The model under review builds one solid part; all positions refer to its coordinate system, in mm. A direction names the side the tool comes from. Coordinates: 2 decimals unless noted, no trailing zeros. Loops run counter-clockwise (first coordinate to the right, second up) from the corner with the lowest first, then second, coordinate; pieces in that order, holes last. Notation, with made-up numbers: (84.25, 60) -> (103.25, 60) arc R5 ccw to (103.25, 66) -> close; hole circle Ø6 at (9, -7.5). An arc over 180 degrees is marked (long way). One line per question, with ' | ' between items. Start each with the question number.
from build123d import *

# Parameters (mm, degrees)
F0_W        = 110
F0_H        = 110
F0_R        = 7
F0_R_2      = 6.6
F0_R_3      = 4.5
F0_R_4      = 5.5
F1_DEPTH    = 20
F2_DEPTH    = 20.001
F3_DEPTH    = 8
F4_DEPTH    = 9.4
F5_SIZE     = 1
F6_T1_DEPTH = 133.7168298797
F6_T3_DEPTH = 133.7168298797
F7_SIZE     = 0.5


# Not quite as in the source:
# - a fillet or chamfer that OpenCascade refuses, or shapes differently, is made with other operations: its cross-section is extruded or revolved along the edge and cut away or added


with BuildPart() as f1:
    # F0 (on Right) → F1 (new body)
    with BuildSketch(Plane.YZ):
        Rectangle(F0_W, F0_H)
        with Locations((-42.4264068712, -42.4264068712)):
            Circle(F0_R, mode=Mode.SUBTRACT)
        with Locations((42.4264068712, -42.4264068712)):
            Circle(F0_R, mode=Mode.SUBTRACT)
        with Locations((-42.4264068712, 42.4264068712)):
            Circle(F0_R, mode=Mode.SUBTRACT)
        Circle(F0_R_2, mode=Mode.SUBTRACT)
        with Locations((42.4264068712, 42.4264068712)):
            Circle(F0_R, mode=Mode.SUBTRACT)
        with Locations((-42.4264068712, 42.4264068712)):
            Circle(F0_R)
        with Locations((-42.4264068712, 42.4264068712)):
            Circle(F0_R_3, mode=Mode.SUBTRACT)
        with Locations((-42.4264068712, -42.4264068712)):
            Circle(F0_R)
        with Locations((-42.4264068712, -42.4264068712)):
            Circle(F0_R_3, mode=Mode.SUBTRACT)
        with Locations((42.4264068712, -42.4264068712)):
            Circle(F0_R)
        with Locations((42.4264068712, -42.4264068712)):
            Circle(F0_R_3, mode=Mode.SUBTRACT)
        with Locations((42.4264068712, 42.4264068712)):
            Circle(F0_R)
        with Locations((42.4264068712, 42.4264068712)):
            Circle(F0_R_3, mode=Mode.SUBTRACT)
        Circle(F0_R_2)
        Circle(F0_R_4, mode=Mode.SUBTRACT)
        Circle(F0_R_4)
        with Locations((-42.4264068712, 42.4264068712)):
            Circle(F0_R_3)
        with Locations((-42.4264068712, -42.4264068712)):
            Circle(F0_R_3)
        with Locations((42.4264068712, -42.4264068712)):
            Circle(F0_R_3)
        with Locations((42.4264068712, 42.4264068712)):
            Circle(F0_R_3)
    extrude(amount=-F1_DEPTH)

    # F0 (on Right) → F2 (cut, through all)
    with BuildSketch(Plane.YZ):
        with Locations((-42.4264068712, 42.4264068712)):
            Circle(F0_R_3)
        with Locations((42.4264068712, -42.4264068712)):
            Circle(F0_R_3)
        with Locations((-42.4264068712, -42.4264068712)):
            Circle(F0_R_3)
        Circle(F0_R_4)
        with Locations((42.4264068712, 42.4264068712)):
            Circle(F0_R_3)
    extrude(amount=-F2_DEPTH, mode=Mode.SUBTRACT)

    # F0 (on Right) → F3 (cut)
    with BuildSketch(Plane.YZ):
        with Locations((-42.4264068712, 42.4264068712)):
            Circle(F0_R)
        with Locations((-42.4264068712, 42.4264068712)):
            Circle(F0_R_3, mode=Mode.SUBTRACT)
        with Locations((42.4264068712, 42.4264068712)):
            Circle(F0_R)
        with Locations((42.4264068712, 42.4264068712)):
            Circle(F0_R_3, mode=Mode.SUBTRACT)
        with Locations((-42.4264068712, -42.4264068712)):
            Circle(F0_R)
        with Locations((-42.4264068712, -42.4264068712)):
            Circle(F0_R_3, mode=Mode.SUBTRACT)
        with Locations((42.4264068712, -42.4264068712)):
            Circle(F0_R)
        with Locations((42.4264068712, -42.4264068712)):
            Circle(F0_R_3, mode=Mode.SUBTRACT)
    extrude(amount=-F3_DEPTH, mode=Mode.SUBTRACT)

    # F0 (on Right) → F4 (cut)
    with BuildSketch(Plane.YZ):
        Circle(F0_R_2)
        Circle(F0_R_4, mode=Mode.SUBTRACT)
    extrude(amount=-F4_DEPTH, mode=Mode.SUBTRACT)

    # F5
    f5_edges = [f1.edges().sort_by_distance(p)[0] for p in [
        (0, -49.426407, 42.426407),
        (0, 35.426407, 42.426407),
        (0, -49.426407, -42.426407),
        (0, 35.426407, -42.426407),
        (-10, 55, -55),
        (-10, 55, 55),
        (-10, -55, 55),
        (-10, -55, -55),
    ]]
    chamfer(f5_edges, length=F5_SIZE)

    # F6: chamfer of 5 on 4 edges, made by hand

    # F6_s2 → F6_t1 (cut)
    with BuildSketch(Plane.XY.offset(-66.8584149398)):
        Polygon((0, -50), (-5, -55), (0, -55), align=None)
        Polygon((-5, 55), (0, 50), (0, 55), align=None)
    extrude(amount=F6_T1_DEPTH, mode=Mode.SUBTRACT)

    # F6_s4 → F6_t3 (cut)
    with BuildSketch(Plane.XZ.offset(-66.8584149398)):
        Polygon((0, 50), (-5, 55), (0, 55), align=None)
        Polygon((0, -50), (-5, -55), (0, -55), align=None)
    extrude(amount=F6_T3_DEPTH, mode=Mode.SUBTRACT)

    # F7
    f7_edges = [f1.edges().sort_by_distance(p)[0] for p in [
        (-20, 37.926407, -42.426407),
        (-20, 37.926407, 42.426407),
        (-20, -46.926407, 42.426407),
        (-20, -46.926407, -42.426407),
        (-20, -5.5, 0),
    ]]
    chamfer(f7_edges, length=F7_SIZE)


solid = f1.part
1) Consider section C-C, the plane y = -42.5. Give the number of separate pieces and of enclosed holes in the cut face, plus the area to 3 significant figures.
2) Machinability: for faces 4 (the face through (-8, 47, 41)), 5 (the face through (-13.67, 41.45, -46.82)), which of the approach directions +Z, -Z, +X, -X, +Y, -Y give a long, thin tool a straight path to every point of the face, cutting with its end or side? Answer none if there is none.
3) Wall thickness on L1, parallel to Z at x = -10, y = 42; L2, parallel to Y at x = -10.5, z = 39; L3, parallel to Y at x = -6.5, z = -40: over which ranges is each line inside the solid? List them lowest first.
4) Insertion check: pin 1 Ø14.5 at (y, z) = (-42.43, 42.43) entering from +X; pin 2 Ø9 at (y, z) = (0, 0) entering from +X; pin 3 Ø7 at (y, z) = (-43.5, 44) entering from +X; pin 4 Ø3 at (x, y) = (-3, 38) entering from +Z. Each pin has a flat end and moves straight along its axis. Give the tip position at first contact, or say it passes through.
5) Consider section A-A, the plane y = 0. Write out the cut boundary in (x, z), plus the area to 3 significant figures.
6) Mouldability with a two-part tool opening along Y and no side actions: class faces 1 (the face through (-4.451, -43.338, -35.486)), 2 (the face through (-12, 55, -1)), 3 (the face through (0, 49, -48)) as +Y half, -Y half, draft (parallel to the pull), parting line (faces both ways), or undercut.
Filled sheet:
1) separate pieces: 3 | enclosed holes: 0 | area: 1,730 mm^2
2) face 4: +X | face 5: +X, -X
3) L1: -55 to -46.91, -37.95 to 37.95, 46.91 to 55 | L2: -55 to -45.34, -39.51 to 39.51, 45.34 to 55 | L3: -55 to -48.99, -35.86 to 35.86, 48.99 to 55
4) pin 1: x = -0.74 | pin 2: through | pin 3: x = -8 | pin 4: z = 54.5
5) outline: (-20, -55) -> (-5, -55) -> (0, -50) -> (0, -6.6) -> (-9.4, -6.6) -> (-9.4, -5.5) -> (-19.5, -5.5) -> (-20, -6) -> close; (-20, 6) -> (-19.5, 5.5) -> (-9.4, 5.5) -> (-9.4, 6.6) -> (0, 6.6) -> (0, 50) -> (-5, 55) -> (-20, 55) -> close | area: 1,930 mm^2
6) face 1: undercut | face 2: +Y half | face 3: draft
